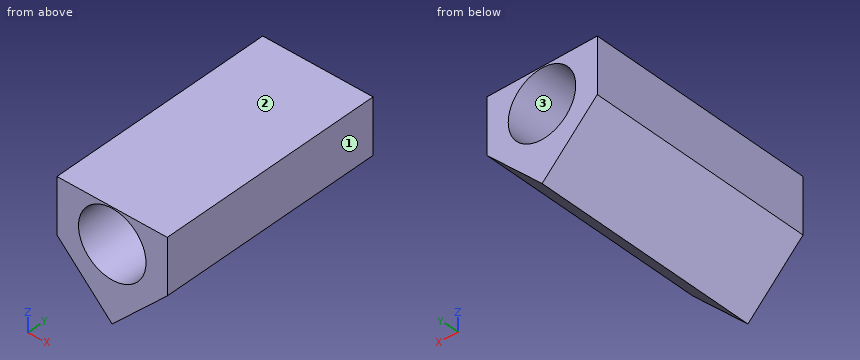
```python
from build123d import *

# Parameters (mm, degrees)
F0_W     = 61.2226556987
F0_H     = 61.2226556987
F1_DEPTH = 127
F2_R     = 18.7364808047
F3_DEPTH = 127.001
F5_DEPTH = 127.001


with BuildPart() as f1:
    # F0 (on Front) → F1 (new body)
    with BuildSketch(Plane.XZ):
        with Locations((-14.1857275739, 9.3327248469)):
            Rectangle(F0_W, F0_H)
    extrude(amount=F1_DEPTH)

    # F2 (on face) → F3 (cut, through all)
    with BuildSketch(Plane.XZ.offset(127)):
        with Locations((-14.1071435064, 20.4563848674)):
            Circle(F2_R)
    extrude(amount=-F3_DEPTH, mode=Mode.SUBTRACT)

    # F4 (on face) → F5 (cut, through all)
    with BuildSketch(Plane(origin=(0, 0, 0), x_dir=(-1, 0, 0), z_dir=(0, 1, 0))):
        Polygon((-16.4256002754, -21.2786030024), (14.1857275739, -21.2786030024), (-16.4256002754, 9.3327248469), align=None)
        Polygon((44.7970554233, 9.3327248469), (14.1857275739, -21.2786030024), (44.7970554233, -21.2786030024), align=None)
    extrude(amount=-F5_DEPTH, mode=Mode.SUBTRACT)


solid = f1.part
```
The listing builds one solid part. Answer for the finished solid, in the listing's coordinates (mm). Face numbers are marked on the shaded views. Round coordinates to 2 decimals unless told otherwise and drop trailing zeros. Loops run counter-clockwise (first coordinate to the right, second up) from the corner with the lowest first, then second, coordinate; pieces in that order, holes last.
Q1. Section D-D, the plane x = -37.5 is taken. Determine the outline of the cut face in (y, z).
Q2. Given pin 1 Ø3 at (y, z) = (-101.5, -1) entering from -X; pin 2 Ø6 at (y, z) = (-111, -15) entering from +X; pin 3 Ø6 at (x, z) = (1.5, 16.5) entering from -Y; pin 4 Ø3 at (y, z) = (-59, -9) entering from -X, each flat-ended and moving along its own axis, determine where each tip first touches the part or whether it passes through.
Q3. Section A-A, the plane z = 16.5 is taken. Determine the outline of the cut face in (x, y).
Q4. Find the intervals of material crossed by line 1 (Z direction, x = -6, y = -29.5); line 2 (X direction, y = -49.5, z = 37); line 3 (Z direction, x = -7.5, y = -113.5), in increasing order.
Q5. Section B-B, the plane x = 0 is taken. Determine the outline of the cut face in (y, z).
Q6. For a pull along Z with two mould halves and no side action, classify the marked faces 1, 2 and 3 as released by +Z, released by -Z, zero draft, split by the parting line, or undercut.
Q7. Section C-C, the plane y = -104.5 is taken. Determine the outline of the cut face in (x, z).
Completed:
1. outline: (-127, 2.04) - (0, 2.04) - (0, 39.94) - (-127, 39.94) - close
2. pin 1: stops at x = -35.96
2. pin 2: stops at x = -4.91
2. pin 3: stops at y = -127
2. pin 4: stops at x = -27.96
3. outline: (-44.8, -127) - (-32.42, -127) - (-32.42, 0) - (-44.8, 0) - close; (4.21, -127) - (16.43, -127) - (16.43, 0) - (4.21, 0) - close
4. line 1: z = -13.09 to 3.56, 37.35 to 39.94
4. line 2: x = -44.8 to -22.9, -5.31 to 16.43
4. line 3: z = -14.59 to 2.92, 37.99 to 39.94
5. outline: (-127, -7.09) - (0, -7.09) - (0, 8.13) - (-127, 8.13) - close; (-127, 32.79) - (0, 32.79) - (0, 39.94) - (-127, 39.94) - close
6. face 1: zero draft
6. face 2: released by +Z
6. face 3: undercut
7. outline: (-44.8, 9.33) - (-14.19, -21.28) - (16.43, 9.33) - (16.43, 39.94) - (-44.8, 39.94) - close; hole circle Ø37.47 at (-14.11, 20.46)
